Verification items for the finished model (mm, model axes). Give positions to 0.01 mm unless a question says otherwise; leave off trailing zeros. Write each loop counter-clockwise with the first axis right and the second up, starting at its lowest first coordinate (ties: lowest second). Pieces come first, ordered by that corner, then holes. Notation, with made-up numbers: (-15.75, 48.5) - (18.25, 48.5) arc R22 cw to (18.25, 81.5) - close; hole circle Ø8 at (16.25, 8). An arc over 180 degrees is marked (long way). Answer as a JSON object with one key per item and string values. Group by question number.
Item 1: Sectioned sample at C-C, the plane z = -1.3. Record the boundary of the cut face in (x, y) (3 decimals).
Item 2: Scan lines: line 1 along X through (y, z) = (113, -2.3); line 2 along Y through (x, z) = (32, -1.2) (3 decimals); line 3 along Y through (x, z) = (19.5, -2.3) (3 decimals). Record each from-to range of solid material in increasing order. Write a range as [from, to].
Item 3: Sectioned sample at B-B, the plane x = 60. Record the boundary of the cut face in (y, z) (3 decimals).
Item 4: Draft check along Y on faces 1 (the face through (40.215, 208.008, -1.565)), 2 (the face through (48, 110, -3.175)), 3 (the face through (40.496, 216.234, -1.565)). Enter one of: +Y half, -Y half, draft (parallel to the pull), parting line (faces both ways), or undercut.
Item 5: Sectioned sample at D-D, the plane x = 40. Count the separate pieces of the cut face and the enclosed holes in it, and give its area (3 significant figures).
Item 6: Sectioned sample at A-A, the plane y = 187.5. Record the boundary of the cut face in (x, z) (3 decimals), and give its area (3 significant figures).
```python
from build123d import *

# Parameters (mm, degrees)
SKETCH1_W           = 10
SKETCH1_H           = 187.325
BOSS_EXTRUDE1_DEPTH = 3.175


with BuildPart() as part:
    # Sketch1 → Boss-Extrude1 (new body)
    with BuildSketch(Plane.XY):
        with BuildLine():
            Line((0, 0), (79.756, 0))
            Line((79.756, 0), (79.756, 200.025))
            ThreePointArc((79.756, 200.025), (39.878, 216.237637896), (0, 200.025))
            Line((0, 200.025), (0, 0))
        make_face()
        with BuildLine():
            Line((17.653, 200.025), (62.103, 200.025))
            ThreePointArc((62.103, 200.025), (39.878, 208.009231637), (17.653, 200.025))
        make_face(mode=Mode.SUBTRACT)
        with Locations((39.878, 100.0125)):
            Rectangle(SKETCH1_W, SKETCH1_H, mode=Mode.SUBTRACT)
    extrude(amount=-BOSS_EXTRUDE1_DEPTH)


solid = part.part
```
Geometry check:
{
 "1": {"outline": "(0, 0) - (79.756, 0) - (79.756, 200.025) arc R57.15 ccw to (0, 200.025) - close; hole (17.653, 200.025) - (62.103, 200.025) arc R34.925 ccw to start; hole (34.878, 6.35) - (44.878, 6.35) - (44.878, 193.675) - (34.878, 193.675) - close"},
 "2": {"line 1": "[0, 34.88], [44.88, 79.76]", "line 2": "[0, 200.025], [207.109, 215.692]", "line 3": "[0, 200.025], [201.448, 212.481]"},
 "3": {"outline": "(0, -3.175) - (200.025, -3.175) - (200.025, 0) - (0, 0) - close; (201.63, -3.175) - (212.578, -3.175) - (212.578, 0) - (201.63, 0) - close"},
 "4": {"face 1": "undercut", "face 2": "draft", "face 3": "+Y half"},
 "5": {"separate pieces": "3", "enclosed holes": "0", "area": "66.4 mm^2"},
 "6": {"outline": "(0, -3.175) - (34.878, -3.175) - (34.878, 0) - (0, 0) - close; (44.878, -3.175) - (79.756, -3.175) - (79.756, 0) - (44.878, 0) - close", "area": "221 mm^2"}
}
